```python
from build123d import *

# Parameters (mm, degrees)
SKETCH1_R           = 12
SKETCH1_R_2         = 1
BOSS_EXTRUDE1_DEPTH = 1.6
SKETCH2_R           = 14.9
SKETCH2_R_2         = 12
BOSS_EXTRUDE2_DEPTH = 1.6
SKETCH3_R           = 1
CUT_EXTRUDE1_DEPTH  = 10


with BuildPart() as part:
    # Sketch1 → Boss-Extrude1 (new body)
    with BuildSketch(Plane.XY):
        with BuildLine():
            Line((-1.5, 16.4), (-1.5, 21.44761059))
            ThreePointArc((-1.5, 21.44761059), (-3.363340998, 21.235299323), (-5.201091386, 20.861415302))
            Line((-5.201091386, 20.861415302), (-3.641293933, 16.060852359))
            ThreePointArc((-3.641293933, 16.060852359), (-4.604353216, 14.170742093), (-6.494463482, 15.133801376))
            Line((-6.494463482, 15.133801376), (-8.054260935, 19.934364319))
            ThreePointArc((-8.054260935, 19.934364319), (-9.760795744, 19.15664027), (-11.39306371, 18.233159334))
            Line((-11.39306371, 18.233159334), (-8.426152646, 14.149556586))
            ThreePointArc((-8.426152646, 14.149556586), (-8.758000259, 12.054353216), (-10.853203629, 12.386200829))
            Line((-10.853203629, 12.386200829), (-13.820114693, 16.469803577))
            ThreePointArc((-13.820114693, 16.469803577), (-15.202795796, 15.202795796), (-16.469803577, 13.820114693))
            Line((-16.469803577, 13.820114693), (-12.386200829, 10.853203629))
            ThreePointArc((-12.386200829, 10.853203629), (-12.054353216, 8.758000259), (-14.149556586, 8.426152646))
            Line((-14.149556586, 8.426152646), (-18.233159334, 11.39306371))
            ThreePointArc((-18.233159334, 11.39306371), (-19.15664027, 9.760795744), (-19.934364319, 8.054260935))
            Line((-19.934364319, 8.054260935), (-15.133801376, 6.494463482))
            ThreePointArc((-15.133801376, 6.494463482), (-14.170742093, 4.604353216), (-16.060852359, 3.641293933))
            Line((-16.060852359, 3.641293933), (-20.861415302, 5.201091386))
            ThreePointArc((-20.861415302, 5.201091386), (-21.235299323, 3.363340998), (-21.44761059, 1.5))
            Line((-21.44761059, 1.5), (-16.4, 1.5))
            ThreePointArc((-16.4, 1.5), (-14.9, 0), (-16.4, -1.5))
            Line((-16.4, -1.5), (-21.44761059, -1.5))
            ThreePointArc((-21.44761059, -1.5), (-21.235299323, -3.363340998), (-20.861415302, -5.201091386))
            Line((-20.861415302, -5.201091386), (-16.060852359, -3.641293933))
            ThreePointArc((-16.060852359, -3.641293933), (-14.170742093, -4.604353216), (-15.133801376, -6.494463482))
            Line((-15.133801376, -6.494463482), (-19.934364319, -8.054260935))
            ThreePointArc((-19.934364319, -8.054260935), (-19.15664027, -9.760795744), (-18.233159334, -11.39306371))
            Line((-18.233159334, -11.39306371), (-14.149556586, -8.426152646))
            ThreePointArc((-14.149556586, -8.426152646), (-12.054353216, -8.758000259), (-12.386200829, -10.853203629))
            Line((-12.386200829, -10.853203629), (-16.469803577, -13.820114693))
            ThreePointArc((-16.469803577, -13.820114693), (-15.202795796, -15.202795796), (-13.820114693, -16.469803577))
            Line((-13.820114693, -16.469803577), (-10.853203629, -12.386200829))
            ThreePointArc((-10.853203629, -12.386200829), (-8.758000259, -12.054353216), (-8.426152646, -14.149556586))
            Line((-8.426152646, -14.149556586), (-11.39306371, -18.233159334))
            ThreePointArc((-11.39306371, -18.233159334), (-9.760795744, -19.15664027), (-8.054260935, -19.934364319))
            Line((-8.054260935, -19.934364319), (-6.494463482, -15.133801376))
            ThreePointArc((-6.494463482, -15.133801376), (-4.604353216, -14.170742093), (-3.641293933, -16.060852359))
            Line((-3.641293933, -16.060852359), (-5.201091386, -20.861415302))
            ThreePointArc((-5.201091386, -20.861415302), (-3.363340998, -21.235299323), (-1.5, -21.44761059))
            Line((-1.5, -21.44761059), (-1.5, -16.4))
            ThreePointArc((-1.5, -16.4), (0, -14.9), (1.5, -16.4))
            Line((1.5, -16.4), (1.5, -21.44761059))
            ThreePointArc((1.5, -21.44761059), (3.363340998, -21.235299323), (5.201091386, -20.861415302))
            Line((5.201091386, -20.861415302), (3.641293933, -16.060852359))
            ThreePointArc((3.641293933, -16.060852359), (4.604353216, -14.170742093), (6.494463482, -15.133801376))
            Line((6.494463482, -15.133801376), (8.054260935, -19.934364319))
            ThreePointArc((8.054260935, -19.934364319), (9.760795744, -19.15664027), (11.39306371, -18.233159334))
            Line((11.39306371, -18.233159334), (8.426152646, -14.149556586))
            ThreePointArc((8.426152646, -14.149556586), (8.758000259, -12.054353216), (10.853203629, -12.386200829))
            Line((10.853203629, -12.386200829), (13.820114693, -16.469803577))
            ThreePointArc((13.820114693, -16.469803577), (15.202795796, -15.202795796), (16.469803577, -13.820114693))
            Line((16.469803577, -13.820114693), (12.386200829, -10.853203629))
            ThreePointArc((12.386200829, -10.853203629), (12.054353216, -8.758000259), (14.149556586, -8.426152646))
            Line((14.149556586, -8.426152646), (18.233159334, -11.39306371))
            ThreePointArc((18.233159334, -11.39306371), (19.15664027, -9.760795744), (19.934364319, -8.054260935))
            Line((19.934364319, -8.054260935), (15.133801376, -6.494463482))
            ThreePointArc((15.133801376, -6.494463482), (14.170742093, -4.604353216), (16.060852359, -3.641293933))
            Line((16.060852359, -3.641293933), (20.861415302, -5.201091386))
            ThreePointArc((20.861415302, -5.201091386), (21.235299323, -3.363340998), (21.44761059, -1.5))
            Line((21.44761059, -1.5), (16.4, -1.5))
            ThreePointArc((16.4, -1.5), (14.9, 0), (16.4, 1.5))
            Line((16.4, 1.5), (21.44761059, 1.5))
            ThreePointArc((21.44761059, 1.5), (21.235299323, 3.363340998), (20.861415302, 5.201091386))
            Line((20.861415302, 5.201091386), (16.060852359, 3.641293933))
            ThreePointArc((16.060852359, 3.641293933), (14.170742093, 4.604353216), (15.133801376, 6.494463482))
            Line((15.133801376, 6.494463482), (19.934364319, 8.054260935))
            ThreePointArc((19.934364319, 8.054260935), (19.15664027, 9.760795744), (18.233159334, 11.39306371))
            Line((18.233159334, 11.39306371), (14.149556586, 8.426152646))
            ThreePointArc((14.149556586, 8.426152646), (12.054353216, 8.758000259), (12.386200829, 10.853203629))
            Line((12.386200829, 10.853203629), (16.469803577, 13.820114693))
            ThreePointArc((16.469803577, 13.820114693), (15.202795796, 15.202795796), (13.820114693, 16.469803577))
            Line((13.820114693, 16.469803577), (10.853203629, 12.386200829))
            ThreePointArc((10.853203629, 12.386200829), (8.758000259, 12.054353216), (8.426152646, 14.149556586))
            Line((8.426152646, 14.149556586), (11.39306371, 18.233159334))
            ThreePointArc((11.39306371, 18.233159334), (9.760795744, 19.15664027), (8.054260935, 19.934364319))
            Line((8.054260935, 19.934364319), (6.494463482, 15.133801376))
            ThreePointArc((6.494463482, 15.133801376), (4.604353216, 14.170742093), (3.641293933, 16.060852359))
            Line((3.641293933, 16.060852359), (5.201091386, 20.861415302))
            ThreePointArc((5.201091386, 20.861415302), (3.363340998, 21.235299323), (1.5, 21.44761059))
            Line((1.5, 21.44761059), (1.5, 16.4))
            ThreePointArc((1.5, 16.4), (0, 14.9), (-1.5, 16.4))
        make_face()
        Circle(SKETCH1_R, mode=Mode.SUBTRACT)
        with Locations((0, 13.5)):
            Circle(SKETCH1_R_2, mode=Mode.SUBTRACT)
        with Locations((13.5, 0)):
            Circle(SKETCH1_R_2, mode=Mode.SUBTRACT)
        with Locations((0, -13.5)):
            Circle(SKETCH1_R_2, mode=Mode.SUBTRACT)
        with Locations((-13.5, 0)):
            Circle(SKETCH1_R_2, mode=Mode.SUBTRACT)
    extrude(amount=BOSS_EXTRUDE1_DEPTH)

    # Sketch2 → Boss-Extrude2 (add)
    with BuildSketch(Plane.XY.offset(1.6)):
        Circle(SKETCH2_R)
        Circle(SKETCH2_R_2, mode=Mode.SUBTRACT)
    extrude(amount=-BOSS_EXTRUDE2_DEPTH)

    # Sketch3 → Cut-Extrude1 (cut)
    with BuildSketch(Plane.XY.offset(1.6)):
        with Locations((9.545941546, 9.545941546)):
            Circle(SKETCH3_R)
        with Locations((9.545941546, -9.545941546)):
            Circle(SKETCH3_R)
        with Locations((-9.545941546, -9.545941546)):
            Circle(SKETCH3_R)
        with Locations((-9.545941546, 9.545941546)):
            Circle(SKETCH3_R)
    extrude(amount=-CUT_EXTRUDE1_DEPTH, mode=Mode.SUBTRACT)


solid = part.part
```
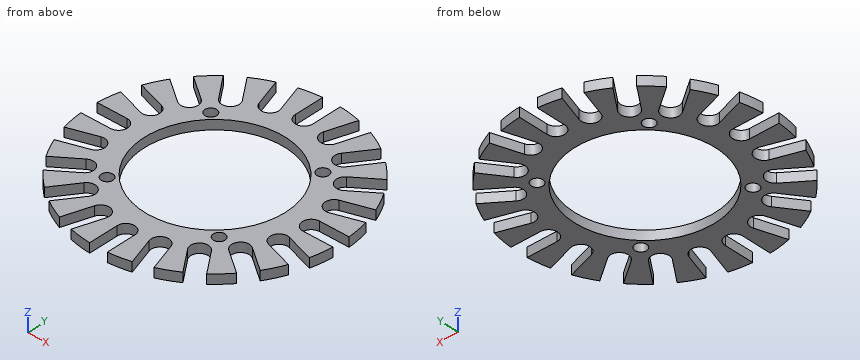
Design review of the part built by this model. Coordinates are the model's own, in mm. Coordinates: 2 decimals unless noted, no trailing zeros. Loops run counter-clockwise (first coordinate to the right, second up) from the corner with the lowest first, then second, coordinate; pieces in that order, holes last.
Q1. We need section B-B on y = 7. State the section outline as (x, z) points.
Reported:
outline: (-16.69, 0) - (-9.75, 0) - (-9.75, 1.6) - (-16.69, 1.6) - close; (9.75, 0) - (16.69, 0) - (16.69, 1.6) - (9.75, 1.6) - close
Q2. To check wall thickness, follow line 1 (Y direction, x = -18, z = 1.4); line 2 (X direction, y = -17, z = 0.3); line 3 (Y direction, x = -10, z = 0.2). State the ranges of each line that lie inside material, in increasing order.
Reported:
line 1: y = -11.22 to -7.43, -4.27 to -1.5, 1.5 to 4.27, 7.43 to 11.22
line 2: x = -10.5 to -7.1, -3.95 to -1.5, 1.5 to 3.95, 7.1 to 10.5
line 3: y = -19.03 to -16.32, -11.81 to -10.44, -8.65 to -6.63, 6.63 to 8.65, 10.44 to 11.81, 16.32 to 19.03
Q3. We need section D-D on x = 17.5. State the section outline as (y, z) points, and give its area (3 significant figures).
Reported:
outline: (-10.86, 0) - (-7.26, 0) - (-7.26, 1.6) - (-10.86, 1.6) - close; (-4.11, 0) - (-1.5, 0) - (-1.5, 1.6) - (-4.11, 1.6) - close; (1.5, 0) - (4.11, 0) - (4.11, 1.6) - (1.5, 1.6) - close; (7.26, 0) - (10.86, 0) - (10.86, 1.6) - (7.26, 1.6) - close
area: 19.9 mm2
Q4. We need section C-C on y = 17. State the section outline as (x, z) points.
Reported:
outline: (-10.5, 0) - (-7.1, 0) - (-7.1, 1.6) - (-10.5, 1.6) - close; (-3.95, 0) - (-1.5, 0) - (-1.5, 1.6) - (-3.95, 1.6) - close; (1.5, 0) - (3.95, 0) - (3.95, 1.6) - (1.5, 1.6) - close; (7.1, 0) - (10.5, 0) - (10.5, 1.6) - (7.1, 1.6) - close
Q5. For pin 1 (0.8 mm diameter, centred on y = 18.5, z = 1, fed in from +X); pin 2 (0.5 mm diameter, centred on y = -20, z = 0.5, fed in from +X); pin 3 (0.5 mm diameter, centred on x = -19, z = 1, fed in from -Y), all flat-tipped, find the tip position at first contact; note any pin that passes through.
Reported:
pin 1: stops at x = 11.39
pin 2: stops at x = 8.5
pin 3: stops at y = -10.52
Q6. We need section A-A on x = 0. State the section outline as (y, z) points.
Reported:
outline: (-14.9, 0) - (-12, 0) - (-12, 1.6) - (-14.9, 1.6) - close; (12, 0) - (14.9, 0) - (14.9, 1.6) - (12, 1.6) - close
